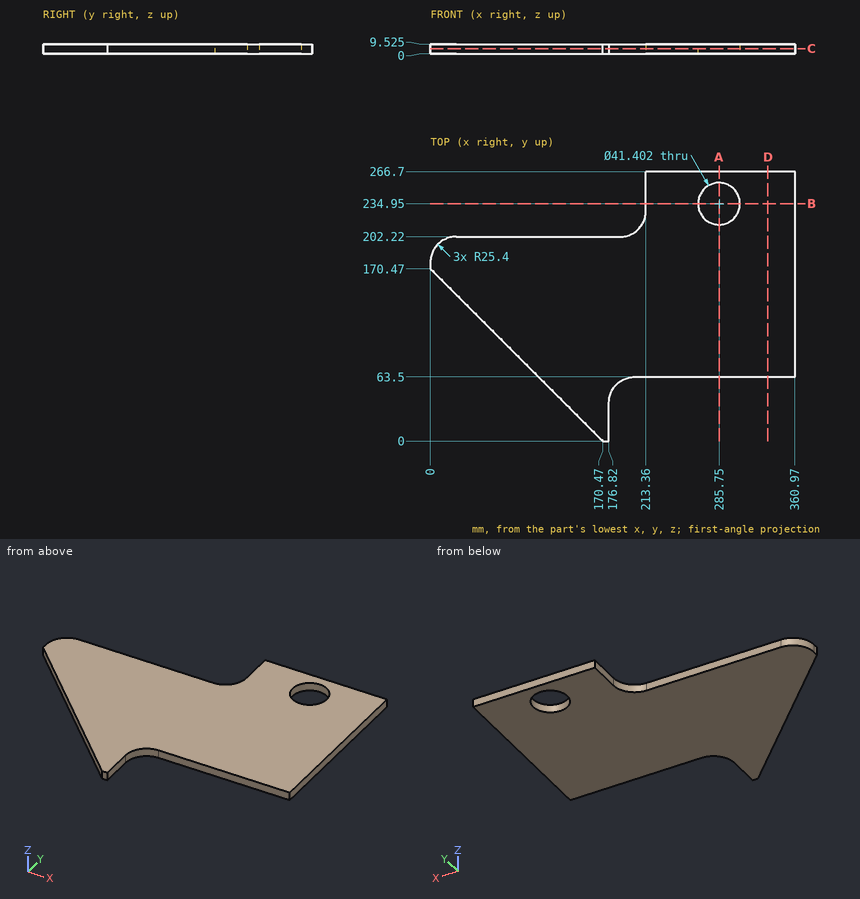
Geometry: see drawing. Coordinates: mm, zero at the bounding-box minimum. Coordinates: 2 decimals unless noted, no trailing zeros. Loops run counter-clockwise (first coordinate to the right, second up) from the corner with the lowest first, then second, coordinate; pieces in that order, holes last.
Q1. Material intervals for line 1 (Y direction, x = 285.75, z = 7); line 2 (Y direction, x = 306.5, z = 1.25); line 3 (X direction, y = 222.5, z = 7), sorted ascending.
Q2. Contact query for flat-ended pins moving along their axis: pin 1 (5 mm diameter, centred on y = 248, z = 7, fed in from -X); pin 2 (2 mm diameter, centred on y = 224, z = 4, fed in from -X); pin 3 (4 mm diameter, centred on x = 157.5, z = 5, fed in from -Y). Output: stop coordinate, or through.
Q3. Cut plane B-B (y = 234.95). Output: boundary loops of the cut face in (x, z) (3 decimals), then the cut area to 3 significant figures.
Q4. Cut plane D-D (x = 334). Output: boundary loops of the cut face in (y, z) (3 decimals).
Q5. Cut plane A-A (x = 285.75). Output: boundary loops of the cut face in (y, z) (3 decimals), then the cut area to 3 significant figures.
Q6. Cut plane C-C (z = 5). Output: boundary loops of the cut face in (x, y).
Working result:
1. line 1: y = 63.5 to 214.25, 255.65 to 266.7
1. line 2: y = 63.5 to 266.7
1. line 3: x = 212.84 to 269.21, 302.29 to 360.97
2. pin 1: stops at x = 213.36
2. pin 2: stops at x = 212.94
2. pin 3: stops at y = 10.97
3. outline: (213.36, 0) - (265.049, 0) - (265.049, 9.525) - (213.36, 9.525) - close; (306.451, 0) - (360.97, 0) - (360.97, 9.525) - (306.451, 9.525) - close
3. area: 1,010 mm2
4. outline: (63.5, 0) - (266.7, 0) - (266.7, 9.525) - (63.5, 9.525) - close
5. outline: (63.5, 0) - (214.249, 0) - (214.249, 9.525) - (63.5, 9.525) - close; (255.651, 0) - (266.7, 0) - (266.7, 9.525) - (255.651, 9.525) - close
5. area: 1,540 mm2
6. outline: (0, 170.47) - (170.47, 0) - (176.82, 0) - (176.82, 38.1) arc R25.4 cw to (202.22, 63.5) - (360.97, 63.5) - (360.97, 266.7) - (213.36, 266.7) - (213.36, 227.62) arc R25.4 cw to (187.96, 202.22) - (25.4, 202.22) arc R25.4 ccw to (0, 176.82) - close; hole circle Ø41.4 at (285.75, 234.95)
